from build123d import *

# Parameters (mm, degrees)
F0_W     = 609.6
F0_H     = 914.4
F1_DEPTH = 19.05
F2_W     = 609.6
F2_H     = 19.05
F3_DEPTH = 9.525


# Not quite as in the source:
# - a length typed as a fraction of an inch, garbled in the dataset ("3 / 203.2 mm" for 3/8 in), is restored


with BuildPart() as f1:
    # F0 (on Front) → F1 (new body)
    with BuildSketch(Plane.XZ):
        with Locations((304.8, 457.2)):
            Rectangle(F0_W, F0_H)
    extrude(amount=F1_DEPTH)

    # F2 (on face) → F3 (cut)
    with BuildSketch(Plane(origin=(0, 0, 0), x_dir=(-1, 0, 0), z_dir=(0, 1, 0))):
        with Locations((-304.8, 79.375)):
            Rectangle(F2_W, F2_H)
        with Locations((-304.8, 454.025)):
            Rectangle(F2_W, F2_H)
        with Locations((-304.8, 828.675)):
            Rectangle(F2_W, F2_H)
    extrude(amount=-F3_DEPTH, mode=Mode.SUBTRACT)


solid = f1.part
The listing builds one solid part. Answer for the finished solid, in the listing's coordinates (mm). A direction names the side the tool comes from. Round coordinates to 2 decimals unless told otherwise and drop trailing zeros. Write each loop counter-clockwise with the first axis right and the second up, starting at its lowest first coordinate (ties: lowest second). Pieces come first, ordered by that corner, then holes. Notation, with made-up numbers: (57, 84) - (99, 84) arc R14 ccw to (99, 105) - close; hole circle Ø4 at (15, 58.5). An arc over 180 degrees is marked (long way). Use a Markdown table: item, result. Add a question column.
1. Consider line 1 (Z direction, x = 142, y = -7.5). Determine where the line is inside the solid, lowest interval first.
2. For a pull along Z with two mould halves and no side action, classify faces 1 (the face through (309, -9.525, 80)), 2 (the face through (301, -9, 0)), 3 (the face through (0, -12, 451)), 4 (the face through (309, -9.525, 454)) as +Z half, -Z half, draft (parallel to the pull), parting line (faces both ways), or undercut.
3. The part is cut by section A-A (y = -4). Write down the section's boundary in (x, z), and give its area (3 significant figures).
4. The part is cut by section C-C (z = 454.5). Write down the section's boundary in (x, y) (3 decimals), and give its area (3 significant figures).
5. A tool of negligible diameter and unlimited length cuts with its end or side. For faces 5 (the face through (309, -9.525, 829)), 6 (the face through (301, 0, 644)), from which of +Z, -Z, +X, -X, +Y, -Y can it reach the whole face along a straight path? Write none if from no direction.
6. The part is cut by section B-B (x = 287). Write down the section's boundary in (y, z) (3 decimals), and give its area (3 significant figures).
7. A flat-ended cylindrical pin translates along its axis: P1, Ø15, axis at x = 375, z = 452.5, coming from the +Y side (3 decimals). Find the tip coordinate at first contact, or state that the pin passes through.
Reported:
| question | item | result |
|---|---|---|
| 1 | line 1 | 0 to 69.85, 88.9 to 444.5, 463.55 to 819.15, 838.2 to 914.4 |
| 2 | face 1 | undercut |
| 2 | face 2 | -Z half |
| 2 | face 3 | draft |
| 2 | face 4 | undercut |
| 3 | outline | (0, 0) - (609.6, 0) - (609.6, 69.85) - (0, 69.85) - close; (0, 88.9) - (609.6, 88.9) - (609.6, 444.5) - (0, 444.5) - close; (0, 463.55) - (609.6, 463.55) - (609.6, 819.15) - (0, 819.15) - close; (0, 838.2) - (609.6, 838.2) - (609.6, 914.4) - (0, 914.4) - close |
| 3 | area | 523,000 mm^2 |
| 4 | outline | (0, -19.05) - (609.6, -19.05) - (609.6, -9.525) - (0, -9.525) - close |
| 4 | area | 5,810 mm^2 |
| 5 | face 5 | +X, -X, +Y |
| 5 | face 6 | +Z, -Z, +X, -X, +Y |
| 6 | outline | (-19.05, 0) - (0, 0) - (0, 69.85) - (-9.525, 69.85) - (-9.525, 88.9) - (0, 88.9) - (0, 444.5) - (-9.525, 444.5) - (-9.525, 463.55) - (0, 463.55) - (0, 819.15) - (-9.525, 819.15) - (-9.525, 838.2) - (0, 838.2) - (0, 914.4) - (-19.05, 914.4) - close |
| 6 | area | 16,900 mm^2 |
| 7 | P1 | y = -9.525 |
